For this review, take the finished solid that the model builds, in its own axes (mm). A direction names the side the tool comes from. Round coordinates to 2 decimals unless told otherwise and drop trailing zeros. Write each loop counter-clockwise with the first axis right and the second up, starting at its lowest first coordinate (ties: lowest second). Pieces come first, ordered by that corner, then holes.
from build123d import *

# Parameters (mm, degrees)
F0_W     = 30.48
F0_H     = 35.56
F0_R     = 1.75
F1_DEPTH = 21.082
F2_R     = 4
F3_DEPTH = 35.56
F4_SIZE  = 1.5875
F5_SIZE  = 0.254
F6_R     = 6.706248
F7_DEPTH = 5.779999
F8_R     = 6.706248
F9_DEPTH = 5.779999


with BuildPart() as f1:
    # F0 (on Top) → F1 (new body)
    with BuildSketch(Plane.XY):
        with Locations((15.24, -17.78)):
            Rectangle(F0_W, F0_H)
        with Locations((6.35, -29.718)):
            Circle(F0_R, mode=Mode.SUBTRACT)
        with Locations((24.13, -29.718)):
            Circle(F0_R, mode=Mode.SUBTRACT)
        with Locations((6.35, -5.842)):
            Circle(F0_R, mode=Mode.SUBTRACT)
        with Locations((24.13, -5.842)):
            Circle(F0_R, mode=Mode.SUBTRACT)
    extrude(amount=F1_DEPTH)

    # F2 (on face) → F3 (cut, through all)
    with BuildSketch(Plane.XZ.offset(35.56)):
        with Locations((15.24, 10.541)):
            Circle(F2_R)
        with BuildLine():
            ThreePointArc((10.31875, 19.862694), (12.704975, 20.772634), (15.24, 21.082))
            Line((15.24, 21.082), (0, 21.082))
            Line((0, 21.082), (0, 3.175))
            Line((0, 3.175), (2.38125, 5.55625))
            Line((2.38125, 5.55625), (2.38125, 19.862694))
            Line((2.38125, 19.862694), (10.31875, 19.862694))
        make_face()
        with BuildLine():
            ThreePointArc((15.24, 21.082), (17.775025, 20.772634), (20.16125, 19.862694))
            Line((20.16125, 19.862694), (28.09875, 19.862694))
            Line((28.09875, 19.862694), (28.09875, 5.55625))
            Line((28.09875, 5.55625), (30.48, 3.175))
            Line((30.48, 3.175), (30.48, 21.082))
            Line((30.48, 21.082), (15.24, 21.082))
        make_face()
    extrude(amount=-F3_DEPTH, mode=Mode.SUBTRACT)

    # F4
    f4_edges = [f1.edges().sort_by_distance(p)[0] for p in [
        (28.09875, -17.78, 19.862694),
        (2.38125, -17.78, 19.862694),
    ]]
    chamfer(f4_edges, length=F4_SIZE)

    # F5
    f5_edges = [f1.edges().sort_by_distance(p)[0] for p in [
        (22.38, -29.718, 19.862694),
        (22.38, -5.842, 19.862694),
        (4.6, -5.842, 19.862694),
        (4.6, -29.718, 19.862694),
    ]]
    chamfer(f5_edges, length=F5_SIZE)

    # F6 (on face) → F7 (cut)
    with BuildSketch(Plane.XZ.offset(35.56)):
        with Locations((15.24, 10.541)):
            Circle(F6_R)
    extrude(amount=-F7_DEPTH, mode=Mode.SUBTRACT)

    # F8 (on face) → F9 (cut)
    with BuildSketch(Plane(origin=(0, 0, 0), x_dir=(-1, 0, 0), z_dir=(0, 1, 0))):
        with Locations((-15.24, 10.541)):
            Circle(F8_R)
    extrude(amount=-F9_DEPTH, mode=Mode.SUBTRACT)


solid = f1.part
(1) We need section D-D, the plane z = 11. Give the boundary of the cut face in (x, y).
Geometry check:
outline: (2.38, -35.56) - (8.55, -35.56) - (8.55, -29.78) - (11.27, -29.78) - (11.27, -5.78) - (8.55, -5.78) - (8.55, 0) - (2.38, 0) - close; (19.21, -29.78) - (21.93, -29.78) - (21.93, -35.56) - (28.1, -35.56) - (28.1, 0) - (21.93, 0) - (21.93, -5.78) - (19.21, -5.78) - close; hole circle Ø3.5 at (6.35, -29.72); hole circle Ø3.5 at (6.35, -5.84); hole circle Ø3.5 at (24.13, -29.72); hole circle Ø3.5 at (24.13, -5.84)
(2) We need section C-C, the plane y = -27. Give the boundary of the cut face in (x, z) (3 decimals), and give its area (3 significant figures).
Geometry check:
outline: (0, 0) - (30.48, 0) - (30.48, 3.175) - (28.099, 5.556) - (28.099, 18.275) - (26.511, 19.863) - (20.161, 19.863) arc R10.541 ccw to (15.24, 21.082) arc R10.541 ccw to (10.319, 19.863) - (3.969, 19.863) - (2.381, 18.275) - (2.381, 5.556) - (0, 3.175) - close; hole circle Ø8 at (15.24, 10.541)
area: 487 mm2
(3) We need section B-B, the plane x = 6.35. Give the boundary of the cut face in (y, z).
Geometry check:
outline: (-35.56, 0) - (-31.47, 0) - (-31.47, 19.61) - (-31.72, 19.86) - (-35.56, 19.86) - close; (-27.97, 0) - (-7.59, 0) - (-7.59, 19.61) - (-7.85, 19.86) - (-27.71, 19.86) - (-27.97, 19.61) - close; (-4.09, 0) - (0, 0) - (0, 19.86) - (-3.84, 19.86) - (-4.09, 19.61) - close
(4) We need section A-A, the plane z = 8. Give the boundary of the cut face in (x, y), and give its area (3 significant figures).
Geometry check:
outline: (2.38, -35.56) - (9.03, -35.56) - (9.03, -29.78) - (12.15, -29.78) - (12.15, -5.78) - (9.03, -5.78) - (9.03, 0) - (2.38, 0) - close; (18.33, -29.78) - (21.45, -29.78) - (21.45, -35.56) - (28.1, -35.56) - (28.1, 0) - (21.45, 0) - (21.45, -5.78) - (18.33, -5.78) - close; hole circle Ø3.5 at (6.35, -29.72); hole circle Ø3.5 at (6.35, -5.84); hole circle Ø3.5 at (24.13, -29.72); hole circle Ø3.5 at (24.13, -5.84)
area: 584 mm2
(5) For pin 1 Ø3 at (x, y) = (6, -9.5) entering from +Z; pin 2 Ø5 at (x, z) = (5, 10.5) entering from +Y; pin 3 Ø3 at (x, z) = (11, 13.5) entering from +Y; pin 4 Ø6.5 at (y, z) = (-18, 14) entering from +X, all flat-tipped, find the tip position at first contact; note any pin that passes through.
Geometry check:
pin 1: stops at z = 19.86
pin 2: stops at y = 0
pin 3: stops at y = -5.78
pin 4: stops at x = 28.1
(6) For line 1 along Y through (x, z) = (6.35, 8.25); line 2 along X through (y, z) = (-7, 15.25); line 3 along Y through (x, z) = (25, 5), list the stretches that pass through material, from the lowest coordinate up.
Geometry check:
line 1: y = -35.56 to -31.47, -27.97 to -7.59, -4.09 to 0
line 2: x = 2.38 to 5.04, 7.66 to 22.82, 25.44 to 28.1
line 3: y = -35.56 to -31.24, -28.2 to -7.36, -4.32 to 0
(7) For faces 1 (the face through (18.33, -32.71, 4.59)), 2 (the face through (28.099, -18, 12)), 3 (the face through (15, -5.78, 6)), list the 3-axis set-ups (+Z, -Z, +X, -X, +Y, -Y) from which the entire face can be reached by the end or side of a thin tool; tool diameter is ignored.
Geometry check:
face 1: -Y
face 2: +Z, +X, +Y, -Y
face 3: +Y
(8) Mouldability with a two-part tool opening along X and no side actions: class faces 4 (the face through (15, -35.56, 3)), 5 (the face through (30.48, -18, 2)), 6 (the face through (15, -29.78, 6)) as pulls with the +X half, pulls with the -X half, needs draft (parallel to the pull), parting line crosses it, or undercut.
Geometry check:
face 4: needs draft
face 5: pulls with the +X half
face 6: undercut
